```python
from build123d import *

# Parameters (mm, degrees)
SKETCH_1_W          = 126.5
SKETCH_1_H          = 82.5
SKETCH_1_R          = 2.1
SKETCH_1_W_2        = 44.684550296
SKETCH_1_H_2        = 47.068057481
EXTRUDE_1_DEPTH     = 4
CUT_EXTRUDE_1_DEPTH = 0.5
FILLET_1_R          = 1


with BuildPart() as part:
    # Эскиз1 → Бобышка-Вытянуть1 (new body)
    with BuildSketch(Plane(origin=(0, 60.645974268, 0), x_dir=(-1, 0, 0), z_dir=(0, -1, 0))):
        with Locations((-64.808980694, -89.523129836)):
            Rectangle(SKETCH_1_W, SKETCH_1_H)
        with Locations(Location((-24.808980694, -59.523129836, 0), (0, 0, 90))):
            Circle(SKETCH_1_R, mode=Mode.SUBTRACT)
        with Locations(Location((-104.808980694, -59.523129836, 0), (0, 0, 90))):
            Circle(SKETCH_1_R, mode=Mode.SUBTRACT)
        with Locations(Location((-24.808980694, -119.523129836, 0), (0, 0, 90))):
            Circle(SKETCH_1_R, mode=Mode.SUBTRACT)
        with Locations(Location((-104.808980694, -119.523129836, 0), (0, 0, 90))):
            Circle(SKETCH_1_R, mode=Mode.SUBTRACT)
        with Locations((-64.808980694, -89.523129837)):
            Rectangle(SKETCH_1_W_2, SKETCH_1_H_2, mode=Mode.SUBTRACT)
    extrude(amount=EXTRUDE_1_DEPTH)

    # Эскиз3 → Вырез-Вытянуть1 (cut)
    with BuildSketch(Plane(origin=(0, 56.645974268, 0), x_dir=(-1, 0, 0), z_dir=(0, -1, 0))):
        Polygon((-59.808980694, -57.523129836), (-32.808980694, -57.523129836), (-32.808980694, -84.523129836), (-12.808980694, -84.523129836), (-12.808980694, -94.523129836), (-32.808980694, -94.523129836), (-32.808980694, -121.523129836), (-59.808980694, -121.523129836), (-59.808980694, -130.773129836), (-69.808980694, -130.773129836), (-69.808980694, -121.523129836), (-96.808980694, -121.523129836), (-96.808980694, -94.523129836), (-116.808980694, -94.523129836), (-116.808980694, -84.523129836), (-96.808980694, -84.523129836), (-96.808980694, -57.523129836), (-69.808980694, -57.523129836), (-69.808980694, -48.273129836), (-59.808980694, -48.273129836), align=None)
    extrude(amount=-CUT_EXTRUDE_1_DEPTH, mode=Mode.SUBTRACT)

    # Скругление1
    fillet_1_edges = [part.edges().sort_by_distance(p)[0] for p in [
        (64.808980694, 57.145974268, 130.773129836),
        (64.808980694, 57.145974268, 48.273129836),
    ]]
    fillet(fillet_1_edges, radius=FILLET_1_R)


solid = part.part
```
Source: CAD feature listing. Evaluate the final solid. Frame: model axes, mm. A direction names the side the tool comes from. Give positions to 0.01 mm unless a question says otherwise; leave off trailing zeros. Loops run counter-clockwise (first coordinate to the right, second up) from the corner with the lowest first, then second, coordinate; pieces in that order, holes last. Notation, with made-up numbers: (84, 16.25) -> (91, 16.25) arc R32 ccw to (91, 51.25) -> close; hole circle Ø8 at (-36.75, 74). An arc over 180 degrees is marked (long way). Use a Markdown table: item, result. Add a question column.
(1) Section query A-A (z = 103). Output: boundary loops of the cut face in (x, y), then the cut area to 3 significant figures.
(2) Section query C-C (x = 110.5). Output: boundary loops of the cut face in (y, z), then the cut area to 3 significant figures.
(3) Section query B-B (x = 48.5). Output: boundary loops of the cut face in (y, z).
(4) First-contact query: pin 1 Ø2.5 at (x, z) = (24.81, 59.52) entering from +Y; pin 2 Ø3 at (x, z) = (39.5, 97) entering from -Y. Flat tips, straight axial feed; report the tip coordinate or a pass-through.
(5) Ray query, line 1 (Z direction, x = 24.5, y = 58.7); line 2 (X direction, y = 57.8, z = 92); line 3 (Z direction, x = 70.5, y = 60.2). Return the intervals inside material, ascending.
(6) Section query D-D (y = 59.25). Output: boundary loops of the cut face in (x, z), then the cut area to 3 significant figures.
(7) Pull-direction query (Z, two-part tool) for faces 1 (the face through (66, 59, 130.773)), 2 (the face through (102.76, 58.67, 119.98)), 3 (the face through (1.559, 59, 90)); classes: +Z half, -Z half, draft (parallel to the pull), parting line (faces both ways), or undercut.
(8) Access query for faces 4 (the face through (128.059, 59, 90)), 5 (the face through (65, 59, 113.057)). Directions: +Z, -Z, +X, -X, +Y, -Y. A direction counts if a zero-diameter tool reaches every point of the face in a straight line with its end or side. Return the directions, or none.
Checked values:
| question | item | result |
|---|---|---|
| 1 | outline | (1.56, 56.65) -> (32.81, 56.65) -> (32.81, 57.15) -> (42.47, 57.15) -> (42.47, 60.65) -> (1.56, 60.65) -> close; (87.15, 57.15) -> (96.81, 57.15) -> (96.81, 56.65) -> (128.06, 56.65) -> (128.06, 60.65) -> (87.15, 60.65) -> close |
| 1 | area | 318 mm^2 |
| 2 | outline | (56.65, 48.27) -> (60.65, 48.27) -> (60.65, 130.77) -> (56.65, 130.77) -> (56.65, 94.52) -> (57.15, 94.52) -> (57.15, 84.52) -> (56.65, 84.52) -> close |
| 2 | area | 325 mm^2 |
| 3 | outline | (56.65, 48.27) -> (60.65, 48.27) -> (60.65, 65.99) -> (57.15, 65.99) -> (57.15, 57.52) -> (56.65, 57.52) -> close; (56.65, 121.52) -> (57.15, 121.52) -> (57.15, 113.06) -> (60.65, 113.06) -> (60.65, 130.77) -> (56.65, 130.77) -> close |
| 4 | pin 1 | through |
| 4 | pin 2 | y = 57.15 |
| 5 | line 1 | 48.27 to 57.45, 61.6 to 117.45, 121.6 to 130.77 |
| 5 | line 2 | 1.56 to 42.47, 87.15 to 128.06 |
| 5 | line 3 | 48.27 to 65.99, 113.06 to 130.77 |
| 6 | outline | (1.56, 48.27) -> (128.06, 48.27) -> (128.06, 130.77) -> (1.56, 130.77) -> close; hole circle Ø4.2 at (24.81, 59.52); hole circle Ø4.2 at (24.81, 119.52); hole (42.47, 65.99) -> (87.15, 65.99) -> (87.15, 113.06) -> (42.47, 113.06) -> close; hole circle Ø4.2 at (104.81, 59.52); hole circle Ø4.2 at (104.81, 119.52) |
| 6 | area | 8,280 mm^2 |
| 7 | face 1 | +Z half |
| 7 | face 2 | undercut |
| 7 | face 3 | draft |
| 8 | face 4 | +Z, -Z, +X, +Y, -Y |
| 8 | face 5 | +Y, -Y |
